Geometry: final body of the model. Coordinates: model frame, mm. Face numbers are marked on the shaded views. A direction names the side the tool comes from. Round coordinates to 2 decimals unless told otherwise and drop trailing zeros. Loops run counter-clockwise (first coordinate to the right, second up) from the corner with the lowest first, then second, coordinate; pieces in that order, holes last. Notation, with made-up numbers: M -32,57.25 L -13,57.25 A14 ccw -13,70.25 Z; hole C 32.5,56 d11. An arc over 180 degrees is marked long. Answer as a JSON object with one key per item and string values.
from build123d import *

# Parameters (mm, degrees)
F0_W     = 50
F0_H     = 50
F1_DEPTH = 9
F2_W     = 23
F2_H     = 26
F3_DEPTH = 6.5
F4_R     = 5


with BuildPart() as f1:
    # F0 (on Top) → F1 (new body)
    with BuildSketch(Plane.XY):
        Rectangle(F0_W, F0_H)
    extrude(amount=F1_DEPTH)

    # F2 (on face) → F3 (cut)
    with BuildSketch(Plane.XY.offset(9)):
        Rectangle(F2_W, F2_H)
    extrude(amount=-F3_DEPTH, mode=Mode.SUBTRACT)

    # F4
    f4_edges = [f1.edges().sort_by_distance(p)[0] for p in [
        (-25, -25, 4.5),
        (25, -25, 4.5),
        (0, 25, 9),
        (-25, 0, 9),
        (25, 0, 9),
        (0, -25, 9),
        (-25, 25, 4.5),
        (25, 25, 4.5),
    ]]
    fillet(f4_edges, radius=F4_R)


solid = f1.part
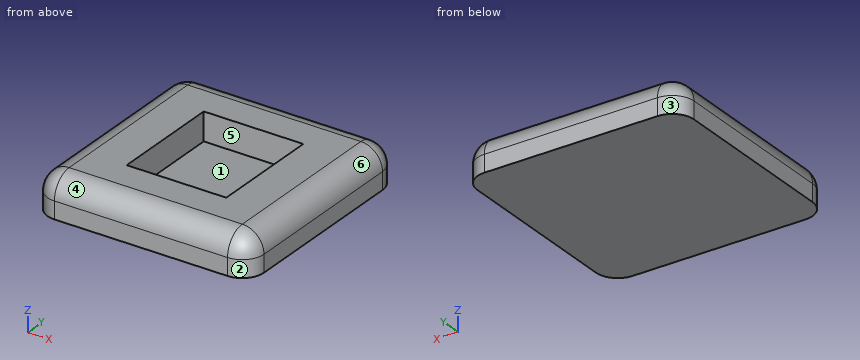
1) Section query D-D (y = 16.5). Return the cut outline in (x, z).
Results:
{"outline": "M -25,0 L 25,0 L 25,4 A5 ccw 20,9 L -20,9 A5 ccw -25,4 Z"}
2) Pin query (flat end, axial travel): P1, Ø2, axis at x = 5, z = 7, coming from the +Y side; P2, Ø2, axis at x = 2, z = 8, coming from the +Y side; P3, Ø18.5, axis at x = -1, y = -1, coming from the +Z side. Return the tip coordinate at first contact, or that it passes through.
Results:
{"P1": "y = 24.58", "P2": "y = 24", "P3": "z = 2.5"}
3) Pull-direction query (X, two-part tool) for the marked faces 3, 4, 5 and 6; classes: +X half, -X half, draft (parallel to the pull), parting line (faces both ways), or undercut.
Results:
{"face 3": "-X half", "face 4": "draft", "face 5": "undercut", "face 6": "+X half"}
4) Ray query, line 1 (Y direction, x = -1.5, z = 3); line 2 (Z direction, x = -4, y = -7); line 3 (Y direction, x = 5, z = 7). Return the intervals inside material, ascending.
Results:
{"line 1": "-25 to -13, 13 to 25", "line 2": "0 to 2.5", "line 3": "-24 to -13, 13 to 24"}
5) Reachability of the marked faces 1 and 2 from +Z, -Z, +X, -X, +Y, -Y: full face, straight path, thin tool, end or side. Return the list, or none.
Results:
{"face 1": "+Z", "face 2": "+Z, -Z, +X, -Y"}
6) Section query C-C (x = 7). Return the cut outline in (y, z).
Results:
{"outline": "M -25,0 L 25,0 L 25,4 A5 ccw 20,9 L 13,9 L 13,2.5 L -13,2.5 L -13,9 L -20,9 A5 ccw -25,4 Z"}
7) Section query B-B (y = 11). Return the cut outline in (x, z), and give its area (3 significant figures).
Results:
{"outline": "M -25,0 L 25,0 L 25,4 A5 ccw 20,9 L 11.5,9 L 11.5,2.5 L -11.5,2.5 L -11.5,9 L -20,9 A5 ccw -25,4 Z", "area": "290 mm2"}
8) Section query A-A (z = 5.25). Return the cut outline in (x, y), and give its area (3 significant figures).
Results:
{"outline": "M -24.84,-20 A4.84 ccw -20,-24.84 L 20,-24.84 A4.84 ccw 24.84,-20 L 24.84,20 A4.84 ccw 20,24.84 L -20,24.84 A4.84 ccw -24.84,20 Z; hole M -11.5,-13 L 11.5,-13 L 11.5,13 L -11.5,13 Z", "area": "1,850 mm2"}
